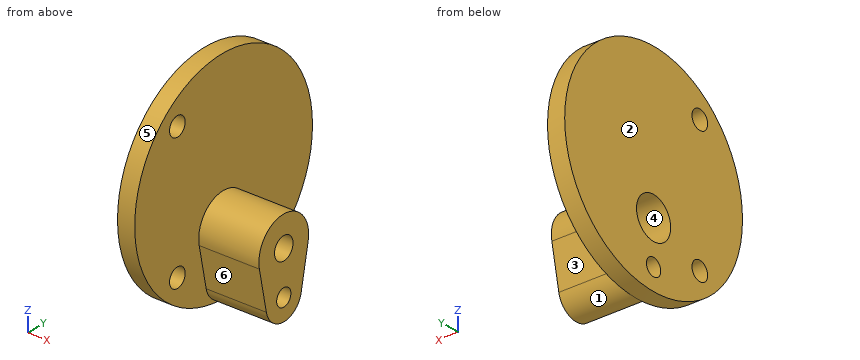
Autodesk Inventor part; units mm, degrees
ref_plane "YZ Plane" through (0, 0, 0) normal (1, 0, 0) x (0, 1, 0)
ref_plane "XZ Plane" through (0, 0, 0) normal (0, 1, 0) x (-1, 0, 0)
ref_plane "XY Plane" through (0, 0, 0) normal (0, 0, 1) x (1, 0, 0)
sketch "スケッチ1" plane through (0, 0, 0) normal (1, 0, 0) x (0, 1, 0)
  circle A0 centre (0, 0) radius 10
  circle A1 centre (0, 0) radius 12.5
  circle A2 centre (0, -5) radius 1.3
  circle A3 centre (0, -10) radius 1
  circle A4 centre (0, -5) radius 3.5
  circle A5 centre (0, -10) radius 2.5
  circle A6 centre (-6.5, 7.7) radius 1.1
  circle A7 centre (-6.5, -7.7) radius 1.1
  line L0 (-6.5, 7.7) -> (-6.5, -7.7)
  line L1 (0, -5) -> (0, -10)
  line L2 (3.5006, -5.3506) -> (2.4495, -10.5)
  line L3 (-3.6097, -4.8161) -> (-2.4495, -10.5)
  dimension "d0" = 20
  dimension "d1" = 25
  dimension "d2" = 2.6
  dimension "d3" = 2
  dimension "d4" = 5
  dimension "d5" = 7
  dimension "d6" = 5
  dimension "d7" = 2.2
  dimension "d8" = 2.2
  dimension "d9" = 15.4
  dimension "d10" = 7.7
  dimension "d12" = 10
  dimension "d13" = 0
  dimension "d14" = 6.5
  dimension "d15" = 3.5
  dimension "d16" = 3.5
extrude "押し出し1" add sketch "スケッチ1" against normal blind 2 contours A0 L2 A4 L3 A7 L0 A6 | A1 | L2 A5 A0 | A0 A5 A4 L2 | A6 L0 A7 A0 | A5 A0 A3 | A0 A3 L1 A4 A5 | A4 A5 | A4 L1 A5 | A3 A0 A5 A4 L1 | A4 A5 L1 | A4 A5 A0 L3 | L3 A0 A5
sketch "スケッチ2" plane through (0, 0, 0) normal (1, 0, 0) x (0, 0, -1)
  circle A0 centre (5, 0) radius 1.3
  circle A1 centre (5, 0) radius 1.3
  circle A2 centre (5, 0) radius 3.5
  circle A3 centre (10, 0) radius 1
  circle A4 centre (10, 0) radius 1
  circle A5 centre (10, 0) radius 2.5
  line L0 (10.9311, 2.3615) -> (5.7, 3.4293)
  line L1 (5.0718, -3.5575) -> (10.5, -2.4495)
  point P0 (0, 0)
  point P1 (5.7, -3.4293)
  point P2 (10.5, 2.4495)
  dimension "d19" = 7
  dimension "d20" = 5
  dimension "d21" = 2.5
  dimension "d22" = 3.5
extrude "押し出し2" add sketch "スケッチ2" along normal blind 7
sketch "スケッチ3" plane through (-2, 0, 0) normal (-1, 0, 0) x (0, 0, 1)
  circle A0 centre (-5, 0) radius 1.3
  circle A1 centre (-5, 0) radius 1.3
  circle A2 centre (-5, 0) radius 2.4
  point P0 (0, 0)
  dimension "d25" = 4.8
extrude "押し出し3" cut sketch "スケッチ3" against normal blind 5
sketch "スケッチ5" plane through (-2, 0, 0) normal (-1, 0, 0) x (0, 0, 1)
  circle A0 centre (0, 0) radius 12.5
  point P0 (-12.5, 0)
ref_plane "作業平面2" through (-2, 0, -12.5) normal (0, 0, -1) x (-1, 0, 0)
equation "\"d8\" = d7"
equation "\"d15\" = 0.5 * d5"
equation "\"d16\" = d15"
properties part number "RSFF_mount_1_clearance"
Could you check a few things on this model? Use its own coordinates, in mm. Face numbers are marked on the shaded views. A direction names the side the tool comes from. Give positions to 0.01 mm unless a question says otherwise; leave off trailing zeros. Write each loop counter-clockwise with the first axis right and the second up, starting at its lowest first coordinate (ties: lowest second). Pieces come first, ordered by that corner, then holes. Notation, with made-up numbers: (62.5, 39) -> (95.5, 39) arc R5 ccw to (95.5, 45) -> close; hole circle Ø9 at (28, 85.5). An arc over 180 degrees is marked (long way). Answer as CSV lines item,"result". Start each with the question number.
(1) I'm going to push flat-ended pins straight in: pin 1 Ø6 at (y, z) = (8, -7) entering from +X; pin 2 Ø1.5 at (x, z) = (-1, -9) entering from +Y. Where does each tip first touch, or does it pass through?
(2) If we section it at D-D, the plane y = 10: Write out the boundary of the cut face in (x, z), and give its area (3 significant figures).
(3) Please list where these lines run through material, in increasing order: line 1 (Y direction, x = 5.9, z = -5); line 2 (Y direction, x = 0.35, z = -5); line 3 (Z direction, x = -1.55, y = -6.5).
(4) Which directions (+Z, -Z, +X, -X, +Y, -Y) give clear straight access to the entire face, cutting with the end or side of a thin tool? Please do the marked faces 1, 2 and 3.
(5) If we section it at B-B, the plane y = -6.5: Write out the boundary of the cut face in (x, z), and give its area (3 significant figures).
(6) If we mould it in two halves opening along Z, with no side actions, what happens to the marked faces 4, 5 and 6? For each: +Z half, -Z half, draft (parallel to the pull), parting line (faces both ways), or undercut.
(7) If we section it at A-A, the plane z = -5: Write out the boundary of the cut face in (x, y).
(8) If we section it at C-C, the plane x = 2.5: Write out the boundary of the cut face in (y, z), and give its area (3 significant figures).
Answer list:
1,pin 1,"x = 0"
1,pin 2,"y = 9.39"
2,outline,"(-2, -7.5) -> (0, -7.5) -> (0, 7.5) -> (-2, 7.5) -> close"
2,area,"30.0 mm^2"
3,line 1,"-3.5 to -1.3, 1.3 to 3.5"
3,line 2,"-3.5 to -2.4, 2.4 to 3.5"
3,line 3,"-10.68 to -8.8, -6.6 to 6.6, 8.8 to 10.68"
4,face 1,"-Z, +X"
4,face 2,"+Z, -Z, -X, +Y, -Y"
4,face 3,"-Z, +X, +Y"
5,outline,"(-2, -10.68) -> (0, -10.68) -> (0, -8.8) -> (-2, -8.8) -> close; (-2, -6.6) -> (0, -6.6) -> (0, 6.6) -> (-2, 6.6) -> close; (-2, 8.8) -> (0, 8.8) -> (0, 10.68) -> (-2, 10.68) -> close"
5,area,"33.9 mm^2"
6,face 4,"undercut"
6,face 5,"parting line"
6,face 6,"-Z half"
7,outline,"(-2, -11.46) -> (0, -11.46) -> (0, -3.5) -> (7, -3.5) -> (7, -1.3) -> (3, -1.3) -> (3, -2.4) -> (-2, -2.4) -> close; (-2, 2.4) -> (3, 2.4) -> (3, 1.3) -> (7, 1.3) -> (7, 3.5) -> (0, 3.5) -> (0, 11.46) -> (-2, 11.46) -> close"
8,outline,"(-3.43, -5.7) -> (-2.45, -10.5) arc R2.5 ccw to (2.45, -10.5) -> (3.43, -5.7) arc R3.5 ccw (long way) to start; hole circle Ø4.8 at (0, -5); hole circle Ø2 at (0, -10)"
8,area,"38.4 mm^2"
